```python
from build123d import *

# Parameters (mm, degrees)
SKETCH1_R           = 6.5
BOSS_EXTRUDE1_DEPTH = 5
CHAMFER1_SIZE       = 0.5
CHAMFER2_SIZE       = 0.5
SKETCH2_R           = 6.5
CUT_EXTRUDE1_DEPTH  = 6
CUT_EXTRUDE2_DEPTH  = 10


with BuildPart() as part:
    # Sketch1 → Boss-Extrude1 (new body)
    with BuildSketch(Plane.XY):
        with BuildLine():
            Line((6.92820323, -58), (53.693575035, 23))
            ThreePointArc((53.693575035, 23), (53.693575035, 31), (46.765371804, 35))
            Line((46.765371804, 35), (-46.765371804, 35))
            ThreePointArc((-46.765371804, 35), (-53.693575035, 31), (-53.693575035, 23))
            Line((-53.693575035, 23), (-6.92820323, -58))
            ThreePointArc((-6.92820323, -58), (0, -62), (6.92820323, -58))
        make_face()
        with Locations((-44.929397948, 25.94)):
            Circle(SKETCH1_R, mode=Mode.SUBTRACT)
        with Locations((44.929397948, 25.94)):
            Circle(SKETCH1_R, mode=Mode.SUBTRACT)
        with Locations((0, -51.88)):
            Circle(SKETCH1_R, mode=Mode.SUBTRACT)
    extrude(amount=-BOSS_EXTRUDE1_DEPTH)

    # Chamfer1
    chamfer1_edges = [part.edges().sort_by_distance(p)[0] for p in [
        (0, 35, 0),
        (53.693575035, 31, 0),
        (30.310889132, -17.5, 0),
        (0, -62, 0),
        (-30.310889132, -17.5, 0),
        (-53.693575035, 31, 0),
    ]]
    chamfer(chamfer1_edges, length=CHAMFER1_SIZE)

    # Chamfer2
    chamfer2_edges = [part.edges().sort_by_distance(p)[0] for p in [
        (0, -62, -5),
        (30.310889132, -17.5, -5),
        (53.693575035, 31, -5),
        (0, 35, -5),
        (-53.693575035, 31, -5),
        (-30.310889132, -17.5, -5),
    ]]
    chamfer(chamfer2_edges, length=CHAMFER2_SIZE)

    # Sketch2 → Cut-Extrude1 (cut, through all)
    with BuildSketch(Plane.XY):
        Circle(SKETCH2_R)
    extrude(amount=-CUT_EXTRUDE1_DEPTH, mode=Mode.SUBTRACT)

    # Sketch3 → Cut-Extrude2 (cut)
    with BuildSketch(Plane.XY):
        Polygon((-1.5, 6.5), (-1.5, 7.9), (1.5, 7.9), (1.5, 6.5), (1.5, 6.224814872), (-1.5, 6.224814872), align=None)
    extrude(amount=-CUT_EXTRUDE2_DEPTH, mode=Mode.SUBTRACT)


solid = part.part
```
Source: CAD feature listing. Evaluate the final solid. Frame: model axes, mm. A direction names the side the tool comes from. Give positions to 0.01 mm unless a question says otherwise; leave off trailing zeros. Write each loop counter-clockwise with the first axis right and the second up, starting at its lowest first coordinate (ties: lowest second). Pieces come first, ordered by that corner, then holes.
1. Pull-direction query (Y, two-part tool) for faces 3 (the face through (-38.73, 27.89, -2.46)), 4 (the face through (53.433, 30.72, -4.865)), 5 (the face through (-1, 9, -5)), 6 (the face through (0, -62, -2)); classes: +Y half, -Y half, draft (parallel to the pull), parting line (faces both ways), or undercut.
2. Section query C-C (y = -51.88). Return the cut outline in (x, z).
3. First-contact query: pin 1 (1.3 mm diameter, centred on y = 7, z = -3.5, fed in from -X); pin 2 (0.5 mm diameter, centred on y = 6.5, z = -3, fed in from +X). Flat tips, straight axial feed; report the tip coordinate or a pass-through.
4. Material intervals for line 1 along Y through (x, z) = (-1, -2.5); line 2 along X through (y, z) = (4, -1.9); line 3 along X through (y, z) = (-49.5, -4.45), sorted ascending.
5. Access query for faces 1 (the face through (0, 7.9, -2)), 2 (the face through (53.75, 30.9, -2.47)). Directions: +Z, -Z, +X, -X, +Y, -Y. A direction counts if a zero-diameter tool reaches every point of the face in a straight line with its end or side. Return the directions, or none.
6. Section query B-B (z = -2.55). Return the cut outline in (x, y), then the cut area to 3 significant figures.
7. Section query D-D (x = 40). Return the cut outline in (y, z), then the cut area to 3 significant figures.
8. Section query A-A (x = 0). Return the cut outline in (y, z), then the cut area to 4 significant figures.
Output values:
1. face 3: undercut
1. face 4: parting line
1. face 5: draft
1. face 6: -Y half
2. outline: (-10.46, -4.5) - (-9.88, -5) - (-6.5, -5) - (-6.5, 0) - (-9.88, 0) - (-10.46, -0.5) - close; (6.5, -5) - (9.88, -5) - (10.46, -4.5) - (10.46, -0.5) - (9.88, 0) - (6.5, 0) - close
3. pin 1: stops at x = -44.83
3. pin 2: stops at x = 44.31
4. line 1: y = -61.94 to -58.3, -45.46 to -6.42, 7.9 to 35
4. line 2: x = -42.72 to -5.12, 5.12 to 42.72
4. line 3: x = -11.84 to -6.05, 6.05 to 11.84
5. face 1: +Z, -Z
5. face 2: +Z, -Z, +X
6. outline: (-53.69, 23) - (-6.93, -58) arc R8 ccw to (6.93, -58) - (53.69, 23) arc R8 ccw to (46.77, 35) - (-46.77, 35) arc R8 ccw to start; hole circle Ø13 at (-44.93, 25.94); hole circle Ø13 at (0, -51.88); hole (-1.5, 6.32) arc R6.5 ccw (long way) to (1.5, 6.32) - (1.5, 7.9) - (-1.5, 7.9) - close; hole circle Ø13 at (44.93, 25.94)
6. area: 5,700 mm2
7. outline: (-0.72, -4.5) - (0.28, -5) - (21.7, -5) - (21.7, 0) - (0.28, 0) - (-0.72, -0.5) - close; (30.18, -5) - (34.5, -5) - (35, -4.5) - (35, -0.5) - (34.5, 0) - (30.18, 0) - close
7. area: 135 mm2
8. outline: (-62, -4.5) - (-61.5, -5) - (-58.38, -5) - (-58.38, 0) - (-61.5, 0) - (-62, -0.5) - close; (-45.38, -5) - (-6.5, -5) - (-6.5, 0) - (-45.38, 0) - close; (7.9, -5) - (34.5, -5) - (35, -4.5) - (35, -0.5) - (34.5, 0) - (7.9, 0) - close
8. area: 347.5 mm2
